The model under review builds one solid part; all positions refer to its coordinate system, in mm. A direction names the side the tool comes from. Coordinates: 2 decimals unless noted, no trailing zeros. Write each loop counter-clockwise with the first axis right and the second up, starting at its lowest first coordinate (ties: lowest second). Pieces come first, ordered by that corner, then holes.
```python
from build123d import *

# Parameters (mm, degrees)
SKETCH1_R           = 7.25
BOSS_EXTRUDE1_DEPTH = 5
BOSS_EXTRUDE2_START = 3
BOSS_EXTRUDE2_DEPTH = 3
SKETCH5_W           = 15.42907023
SKETCH5_H           = 3
CUT_EXTRUDE2_DEPTH  = 5
SKETCH7_W           = 3
SKETCH7_H           = 2.5
CUT_EXTRUDE4_DEPTH  = 10
SKETCH8_R           = 2.5
CUT_EXTRUDE5_DEPTH  = 10


with BuildPart() as part:
    # Sketch1 → Boss-Extrude1 (new body)
    with BuildSketch(Plane.XY):
        with BuildLine():
            ThreePointArc((-25.275752705, 5.100552072), (-33.878856947, 10.952155773), (-31.597213811, 21.10344993))
            Line((-31.597213811, 21.10344993), (-18.821461106, 33.062970941))
            ThreePointArc((-18.821461106, 33.062970941), (-15.898396299, 34.913177324), (-12.5, 35.560073083))
            Line((-12.5, 35.560073083), (0, 35.560073083))
            Line((0, 35.560073083), (0, -2))
            Line((0, -2), (-17, -2))
            Line((-17, -2), (-17, 4.350552072))
            ThreePointArc((-17, 4.350552072), (-17.219669914, 4.880882158), (-17.75, 5.100552072))
            Line((-17.75, 5.100552072), (-25.275752705, 5.100552072))
        make_face()
        with Locations((-12.5, 26.310073083)):
            Circle(SKETCH1_R, mode=Mode.SUBTRACT)
        with Locations((-25.275752705, 14.350552072)):
            Circle(SKETCH1_R, mode=Mode.SUBTRACT)
    boss_extrude1 = extrude(amount=BOSS_EXTRUDE1_DEPTH)

    # Mirror1: Boss-Extrude1 across plane
    add(boss_extrude1.mirror(Plane(origin=(0, 0, 0), x_dir=(0, 0, 1), z_dir=(1, 0, 0))))

    # Sketch3 → Boss-Extrude2 (add)
    with BuildSketch(Plane(origin=(0, 0, 0), x_dir=(-1, 0, 0), z_dir=(0, 0, -1)).offset(BOSS_EXTRUDE2_START)):
        with BuildLine():
            Line((31.597213811, 21.10344993), (18.821461106, 33.062970941))
            ThreePointArc((18.821461106, 33.062970941), (15.898396299, 34.913177324), (12.5, 35.560073083))
            Line((12.5, 35.560073083), (-12.5, 35.560073083))
            ThreePointArc((-12.5, 35.560073083), (-15.898396299, 34.913177324), (-18.821461106, 33.062970941))
            Line((-18.821461106, 33.062970941), (-31.597213811, 21.10344993))
            ThreePointArc((-31.597213811, 21.10344993), (-32.028650564, 8.029090966), (-18.954291599, 7.597654213))
            Line((-18.954291599, 7.597654213), (-6.178538894, 19.557175224))
            Line((-6.178538894, 19.557175224), (-1.366802401, 24.061494071))
            ThreePointArc((-1.366802401, 24.061494071), (0, 24.601408047), (1.366802401, 24.061494071))
            Line((1.366802401, 24.061494071), (6.178538894, 19.557175224))
            Line((6.178538894, 19.557175224), (18.954291599, 7.597654213))
            ThreePointArc((18.954291599, 7.597654213), (32.028650564, 8.029090966), (31.597213811, 21.10344993))
        make_face()
    extrude(amount=-BOSS_EXTRUDE2_DEPTH)

    # Sketch5 → Cut-Extrude2 (cut)
    with BuildSketch(Plane.XY.offset(5)):
        Polygon((-12.873838012, 28.014542797), (-28.664096552, 12.764122156), (-26.57998389, 10.606235594), (-10.78972535, 25.856656236), align=None)
        with Locations((0.808061856, 26.310073083)):
            Rectangle(SKETCH5_W, SKETCH5_H)
        Polygon((26.57998389, 10.606235594), (10.78972535, 25.856656236), (12.873838012, 28.014542797), (28.664096552, 12.764122156), align=None)
    extrude(amount=-CUT_EXTRUDE2_DEPTH, mode=Mode.SUBTRACT)

    # Sketch7 → Cut-Extrude4 (cut)
    with BuildSketch(Plane(origin=(-25.285844423, 27.011591434, 0), x_dir=(0.7300430117299187, 0.6834012006313055, 0), z_dir=(-0.6834012006313055, 0.7300430117299187, 0))):
        with Locations((-8.645202113, -1.25)):
            Rectangle(SKETCH7_W, SKETCH7_H)
    cut_extrude4 = extrude(amount=-CUT_EXTRUDE4_DEPTH, mode=Mode.SUBTRACT)

    # Mirror3: Cut-Extrude4 across plane
    add(cut_extrude4.mirror(Plane(origin=(0, 0, 0), x_dir=(0, 0, 1), z_dir=(1, 0, 0))), mode=Mode.SUBTRACT)

    # Sketch8 → Cut-Extrude5 (cut)
    with BuildSketch(Plane.XY.offset(5)):
        with Locations((0, 21)):
            Circle(SKETCH8_R)
    extrude(amount=-CUT_EXTRUDE5_DEPTH, mode=Mode.SUBTRACT)


solid = part.part
```
Item 1: For pin 1 (6 mm diameter, centred on x = 3.5, y = 13, fed in from -Z); pin 2 (1.5 mm diameter, centred on x = 24, z = -2, fed in from +Y); pin 3 (2 mm diameter, centred on y = 20.5, z = 1.5, fed in from -X), all flat-tipped, find the tip position at first contact; note any pin that passes through.
Solved:
pin 1: stops at z = 0
pin 2: stops at y = 28.92
pin 3: stops at x = -32.96
Item 2: To check wall thickness, follow line 1 along Y through (x, z) = (0, 2.95); line 2 along X through (y, z) = (22, 4.75); line 3 along Y through (x, z) = (-12.5, 3.5). State the ranges of each line that lie inside material, in increasing order.
Solved:
line 1: y = -2 to 18.5, 23.5 to 24.81, 27.81 to 35.56
line 2: x = -30.64 to -19.1, -6.67 to -2.29, 2.29 to 6.67, 19.1 to 30.64
line 3: y = -2 to 19.06, 33.56 to 35.56
Item 3: Machinability: for faces 1 (the face through (-31, 20, 2.5)), 2 (the face through (0, 9, 0)), 3 (the face through (-17.781, 19.104, 2.535)), which of the approach directions +Z, -Z, +X, -X, +Y, -Y give a long, thin tool a straight path to every point of the face, cutting with its end or side? Answer none if there is none.
Solved:
face 1: none
face 2: -Z, -Y
face 3: +Z
Item 4: Take a section at C-C, the plane y = 11. Write out the cut boundary in (x, z), plus the area to 3 significant figures.
Solved:
outline: (-33.9, -3) - (-15.32, -3) - (-15.32, 0) - (15.32, 0) - (15.32, -3) - (33.9, -3) - (33.9, 5) - (31.71, 5) - (31.71, 0) - (18.85, 0) - (18.85, 5) - (-18.85, 5) - (-18.85, 0) - (-31.71, 0) - (-31.71, 5) - (-33.9, 5) - close
area: 322 mm2
Item 5: Take a section at D-D, the plane x = -26.5. Write out the cut boundary in (y, z) (3 decimals).
Solved:
outline: (5.182, -3) - (25.875, -3) - (25.875, 5) - (21.496, 5) - (21.496, 0) - (7.205, 0) - (7.205, 5) - (5.182, 5) - close
Item 6: Take a section at B-B, the plane z = 3.5. Write out the cut boundary in (x, y), plus the area to 3 significant figures.
Solved:
outline: (-31.6, 21.1) arc R9.25 ccw to (-25.28, 5.1) - (-17.75, 5.1) arc R0.75 cw to (-17, 4.35) - (-17, -2) - (17, -2) - (17, 4.35) arc R0.75 cw to (17.75, 5.1) - (25.28, 5.1) arc R9.25 ccw to (31.6, 21.1) - (18.82, 33.06) arc R9.25 ccw to (12.5, 35.56) - (-12.5, 35.56) arc R9.25 ccw to (-18.82, 33.06) - close; hole (-20.98, 20.19) arc R7.25 ccw (long way) to (-18.98, 17.95) - (-16.55, 20.3) arc R7.25 ccw to (-5.41, 24.81) - (5.41, 24.81) arc R7.25 ccw to (16.55, 20.3) - (18.98, 17.95) arc R7.25 ccw (long way) to (20.98, 20.19) - (18.64, 22.45) arc R7.25 ccw (long way) to (5.41, 27.81) - (-5.41, 27.81) arc R7.25 ccw (long way) to (-18.64, 22.45) - close; hole circle Ø5 at (0, 21)
area: 1,250 mm2
Item 7: Take a section at A-A, the plane x = 0. Write out the cut boundary in (y, z), plus the area to 3 significant figures.
Solved:
outline: (-2, 0) - (18.5, 0) - (18.5, 5) - (-2, 5) - close; (23.5, 0) - (24.6, 0) - (24.6, -3) - (35.56, -3) - (35.56, 5) - (27.81, 5) - (27.81, 0) - (24.81, 0) - (24.81, 5) - (23.5, 5) - close
area: 181 mm2
Item 8: Mouldability with a two-part tool opening along Z and no side actions: class faces 4 (the face through (-29.775, 21.352, 1.267)), 5 (the face through (0, 24.6, -1.5)), 6 (the face through (0, 17, 5)) as pulls with the +Z half, pulls with the -Z half, needs draft (parallel to the pull), parting line crosses it, or undercut.
Solved:
face 4: undercut
face 5: needs draft
face 6: pulls with the +Z half
